Read the model definition and answer for the solid it produces. Units are mm, in the model's axes. A direction names the side the tool comes from. Give positions to 0.01 mm unless a question says otherwise; leave off trailing zeros. Loops run counter-clockwise (first coordinate to the right, second up) from the corner with the lowest first, then second, coordinate; pieces in that order, holes last.
(1) Find section A-A, the plane z = 0. Write down the section's boundary in (x, y), then the cut area to 3 significant figures.
(2) Find section C-C, the plane z = -4.25. Write down the section's boundary in (x, y).
(3) Determine the mould class of faces 3 (the face through (0, 5.6, 1)), 4 (the face through (-2.44, 3.06, -0.54)), 5 (the face through (-0.488, 2.839, -0.108)) for opening direction X: pulls with the +X half, pulls with the -X half, needs draft (parallel to the pull), parting line crosses it, or undercut.
(4) Straight lines are drawn through the part: probe 1 along X at (y, z) = (3.8, 0); probe 2 along Y at (x, z) = (-2, 3); probe 3 along X at (y, z) = (0.55, 3.5). For each, find the intervals that lie inside material, in ascending order.
(5) Each of these flat-tipped pins is pushed along its axis until it touches: P1, Ø3, axis at x = 5.5, z = 6, coming from the +Y side; P2, Ø1.5, axis at y = 2, z = 2.5, coming from the +X side. Where does it stop, or does it pass through?
(6) Which of the six approach directions +Z, -Z, +X, -X, +Y, -Y give full straight-line access (tool end or side, diameter ignored) to faces 1 (the face through (-2, 0, 0)), 2 (the face through (2, 0.6, 2))?
(7) Find section B-B, the plane x = 0. Write down the section's boundary in (y, z), then the cut area to 3 significant figures.
(8) Find section D-D, the plane x = 4.25. Write down the section's boundary in (y, z).
```python
from build123d import *

# Parameters (mm, degrees)
ESQUISSE1_R             = 8
ESQUISSE1_R_2           = 1
BOSS_EXTRU_1_DEPTH      = 0.6
ESQUISSE2_R             = 2.5
BOSS_EXTRU_2_DEPTH      = 5
ESQUISSE3_R             = 0.5
ENL_V_MAT_EXTRU_1_DEPTH = 5.6
CHANFREIN1_SIZE         = 0.75


with BuildPart() as part:
    # Esquisse1 → Boss.-Extru.1 (new body)
    with BuildSketch(Plane(origin=(0, 0, 0), x_dir=(1, 0, 0), z_dir=(0, 1, 0))):
        with Locations(Location((0, 0, 0), (0, 0, 270))):
            Circle(ESQUISSE1_R)
        with Locations(Location((-4.25, 4.25, 0), (0, 0, 270))):
            Circle(ESQUISSE1_R_2, mode=Mode.SUBTRACT)
        with Locations(Location((4.25, 4.25, 0), (0, 0, 270))):
            Circle(ESQUISSE1_R_2, mode=Mode.SUBTRACT)
        with Locations(Location((4.25, -4.25, 0), (0, 0, 270))):
            Circle(ESQUISSE1_R_2, mode=Mode.SUBTRACT)
        with Locations(Location((-4.25, -4.25, 0), (0, 0, 270))):
            Circle(ESQUISSE1_R_2, mode=Mode.SUBTRACT)
    extrude(amount=BOSS_EXTRU_1_DEPTH)

    # Esquisse2 → Boss.-Extru.2 (add)
    with BuildSketch(Plane(origin=(0, 0.6, 0), x_dir=(1, 0, 0), z_dir=(0, 1, 0))):
        with Locations(Location((0, 0, 0), (0, 0, 270))):
            Circle(ESQUISSE2_R)
    extrude(amount=BOSS_EXTRU_2_DEPTH)

    # Esquisse3 → Enlèv. mat.-Extru.1 (cut)
    with BuildSketch(Plane(origin=(0, 5.6, 0), x_dir=(1, 0, 0), z_dir=(0, 1, 0))):
        with Locations(Location((0, 0, 0), (0, 0, 270))):
            Circle(ESQUISSE3_R)
    extrude(amount=-ENL_V_MAT_EXTRU_1_DEPTH, mode=Mode.SUBTRACT)

    # Chanfrein1
    # the kernel refuses this chamfer: 0.75 mm, written as the material it takes off along each edge
    with BuildSketch(Plane(origin=(4.25, 0, 4.25), x_dir=(0, 0, 1), z_dir=(-1, 0, 0))) as chanfrein1_piece_1:
        Polygon((1 + CHANFREIN1_SIZE, 0), (1, CHANFREIN1_SIZE), (1, 0), align=None)
    revolve(axis=Axis((4.25, 0, 4.25), (0, 1, 0)), mode=Mode.SUBTRACT)
    with BuildSketch(Plane(origin=(-4.25, 0, 4.25), x_dir=(0, 0, 1), z_dir=(-1, 0, 0))) as chanfrein1_piece_2:
        Polygon((1 + CHANFREIN1_SIZE, 0), (1, CHANFREIN1_SIZE), (1, 0), align=None)
    revolve(axis=Axis((-4.25, 0, 4.25), (0, 1, 0)), mode=Mode.SUBTRACT)
    with BuildSketch(Plane(origin=(-4.25, 0, -4.25), x_dir=(0, 0, 1), z_dir=(-1, 0, 0))) as chanfrein1_piece_3:
        Polygon((1 + CHANFREIN1_SIZE, 0), (1, CHANFREIN1_SIZE), (1, 0), align=None)
    revolve(axis=Axis((-4.25, 0, -4.25), (0, 1, 0)), mode=Mode.SUBTRACT)
    with BuildSketch(Plane(origin=(4.25, 0, -4.25), x_dir=(0, 0, 1), z_dir=(-1, 0, 0))) as chanfrein1_piece_4:
        Polygon((1 + CHANFREIN1_SIZE, 0), (1, CHANFREIN1_SIZE), (1, 0), align=None)
    revolve(axis=Axis((4.25, 0, -4.25), (0, 1, 0)), mode=Mode.SUBTRACT)


solid = part.part
```
Entries:
1. outline: (-8, 0) - (-0.5, 0) - (-0.5, 5.6) - (-2.5, 5.6) - (-2.5, 0.6) - (-8, 0.6) - close; (0.5, 0) - (8, 0) - (8, 0.6) - (2.5, 0.6) - (2.5, 5.6) - (0.5, 5.6) - close
1. area: 29.0 mm2
2. outline: (-6.78, 0) - (-6, 0) - (-5.4, 0.6) - (-6.78, 0.6) - close; (-3.1, 0.6) - (-2.5, 0) - (2.5, 0) - (3.1, 0.6) - close; (5.4, 0.6) - (6, 0) - (6.78, 0) - (6.78, 0.6) - close
3. face 3: needs draft
3. face 4: parting line crosses it
3. face 5: undercut
4. probe 1: x = -2.5 to -0.5, 0.5 to 2.5
4. probe 2: y = 0 to 0.6
4. probe 3: x = -7.19 to -5.19, -3.31 to 3.31, 5.19 to 7.19
5. P1: stops at y = 0.6
5. P2: stops at x = 1.79
6. face 1: +Z, -Z, +X, -X, -Y
6. face 2: +Y
7. outline: (0, -8) - (0.6, -8) - (0.6, -2.5) - (5.6, -2.5) - (5.6, -0.5) - (0, -0.5) - close; (0, 0.5) - (5.6, 0.5) - (5.6, 2.5) - (0.6, 2.5) - (0.6, 8) - (0, 8) - close
7. area: 29.0 mm2
8. outline: (0, -6.78) - (0.6, -6.78) - (0.6, -5.4) - (0, -6) - close; (0, -2.5) - (0.6, -3.1) - (0.6, 3.1) - (0, 2.5) - close; (0, 6) - (0.6, 5.4) - (0.6, 6.78) - (0, 6.78) - close
